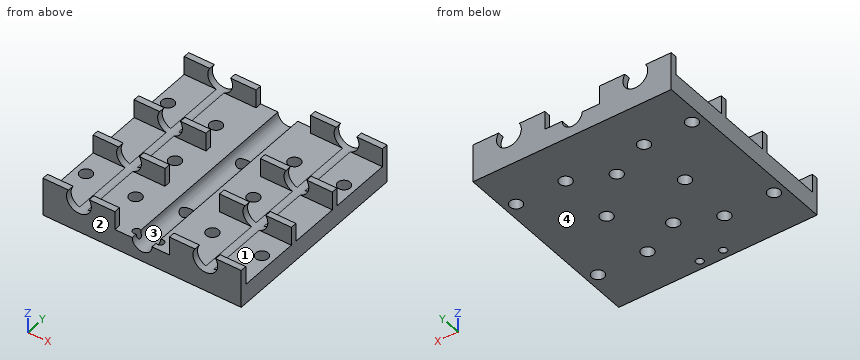
from build123d import *

# Parameters (mm, degrees)
F0_W     = 80
F0_H     = 80
F0_R     = 2.5
F0_R_2   = 1.5
F1_DEPTH = 8
F2_W     = 29
F2_H     = 2.5
F3_DEPTH = 7.5
F5_D     = 10
F7_D     = 8


with BuildPart() as f1:
    # F0 (on Top) → F1 (new body)
    with BuildSketch(Plane.XY):
        Rectangle(F0_W, F0_H)
        with Locations((-35.5, -22.5)):
            Circle(F0_R, mode=Mode.SUBTRACT)
        with Locations((-4.75, -36.5)):
            Circle(F0_R_2, mode=Mode.SUBTRACT)
        with Locations((-15.5, -22.5)):
            Circle(F0_R, mode=Mode.SUBTRACT)
        with Locations((4.75, -36.5)):
            Circle(F0_R_2, mode=Mode.SUBTRACT)
        with Locations((15.5, -22.5)):
            Circle(F0_R, mode=Mode.SUBTRACT)
        with Locations((35.5, -22.5)):
            Circle(F0_R, mode=Mode.SUBTRACT)
        with Locations((0, -15.5)):
            Circle(F0_R, mode=Mode.SUBTRACT)
        with Locations((-16.135083, 0)):
            Circle(F0_R, mode=Mode.SUBTRACT)
        with Locations((-35.5, 22.5)):
            Circle(F0_R, mode=Mode.SUBTRACT)
        with Locations((-16.135083, 22.5)):
            Circle(F0_R, mode=Mode.SUBTRACT)
        with Locations((15.5, 0)):
            Circle(F0_R, mode=Mode.SUBTRACT)
        with Locations((0, 15.5)):
            Circle(F0_R, mode=Mode.SUBTRACT)
        with Locations((15.5, 22.5)):
            Circle(F0_R, mode=Mode.SUBTRACT)
        with Locations((35.5, 22.5)):
            Circle(F0_R, mode=Mode.SUBTRACT)
    extrude(amount=F1_DEPTH)

    # F2 (on face) → F3 (join)
    with BuildSketch(Plane.XY.offset(8)):
        with Locations((-25.5, 38.75)):
            Rectangle(F2_W, F2_H)
        with Locations((25.5, 38.75)):
            Rectangle(F2_W, F2_H)
        with Locations((-25.5, -38.75)):
            Rectangle(F2_W, F2_H)
        with Locations((25.5, -38.75)):
            Rectangle(F2_W, F2_H)
        with Locations((-25.5, -11.25)):
            Rectangle(F2_W, F2_H)
        with Locations((25.5, -11.25)):
            Rectangle(F2_W, F2_H)
        with Locations((-25.5, 11.25)):
            Rectangle(F2_W, F2_H)
        with Locations((25.5, 11.25)):
            Rectangle(F2_W, F2_H)
    extrude(amount=F3_DEPTH)

    # F5 (through all)
    with Locations(Plane(origin=(0, 40, 0), x_dir=(-1, 0, 0), z_dir=(0, 1, 0))):
        with Locations((-25.5, 12.75), (25.5, 12.75)):
            Hole(F5_D / 2)

    # F7 (through all)
    with Locations(Plane(origin=(0, 40, 0), x_dir=(-1, 0, 0), z_dir=(0, 1, 0))):
        with Locations((0, 8)):
            Hole(F7_D / 2)


solid = f1.part
The listing builds one solid part. Answer for the finished solid, in the listing's coordinates (mm). Face numbers are marked on the shaded views. A direction names the side the tool comes from. Round coordinates to 2 decimals unless told otherwise and drop trailing zeros. Write each loop counter-clockwise with the first axis right and the second up, starting at its lowest first coordinate (ties: lowest second). Pieces come first, ordered by that corner, then holes. Notation, with made-up numbers: (47.5, 17) - (66.5, 17) arc R32 cw to (66.5, 44) - close; hole circle Ø6 at (-22, -10). An arc over 180 degrees is marked (long way). Use a Markdown table: item, result. Add a question column.
1. Consider line 1 (Y direction, x = 15.5, z = 4); line 2 (Y direction, x = 18, z = 14.5); line 3 (Y direction, x = 0, z = 2.65). Determine where each line is inside the solid, lowest interval first.
2. The part is cut by section A-A (y = 22.5). Write down the section's boundary in (x, z), and give its area (3 significant figures).
3. The part is cut by section C-C (y = -15.5). Write down the section's boundary in (x, z).
4. The part is cut by section D-D (x = 15.5). Write down the section's boundary in (y, z).
5. A tool of negligible diameter and unlimited length cuts with its end or side. For the marked faces 1 and 2, from which of +Z, -Z, +X, -X, +Y, -Y can it reach the whole face along a straight path? Write none if from no direction.
6. Flat-ended cylindrical pins translate along their axes: P1, Ø3, axis at x = -35.5, y = 22.5, coming from the +Z side; P2, Ø6, axis at x = -16.14, y = 22.5, coming from the +Z side. Find the tip coordinate at first contact, or state that the pin passes through.
7. The part is cut by section B-B (x = 0). Write down the section's boundary in (y, z), and give its area (3 significant figures).
8. For a pull along X with two mould halves and no side action, classify the marked faces 3 and 4 as +X half, -X half, draft (parallel to the pull), parting line (faces both ways), or undercut.
Reported:
| question | item | result |
|---|---|---|
| 1 | line 1 | -40 to -25, -20 to -2.5, 2.5 to 20, 25 to 40 |
| 1 | line 2 | -40 to -37.5, -12.5 to -10, 10 to 12.5, 37.5 to 40 |
| 1 | line 3 | -40 to -18, -13 to 13, 18 to 40 |
| 2 | outline | (-40, 0) - (-38, 0) - (-38, 8) - (-40, 8) - close; (-33, 0) - (-18.64, 0) - (-18.64, 8) - (-23.94, 8) arc R5 cw to (-27.06, 8) - (-33, 8) - close; (-13.64, 0) - (13, 0) - (13, 8) - (4, 8) arc R4 cw to (-4, 8) - (-13.64, 8) - close; (18, 0) - (33, 0) - (33, 8) - (27.06, 8) arc R5 cw to (23.94, 8) - (18, 8) - close; (38, 0) - (40, 0) - (40, 8) - (38, 8) - close |
| 2 | area | 454 mm^2 |
| 3 | outline | (-40, 0) - (-2.5, 0) - (-2.5, 4.88) arc R4 cw to (-4, 8) - (-23.94, 8) arc R5 cw to (-27.06, 8) - (-40, 8) - close; (2.5, 0) - (40, 0) - (40, 8) - (27.06, 8) arc R5 cw to (23.94, 8) - (4, 8) arc R4 cw to (2.5, 4.88) - close |
| 4 | outline | (-40, 0) - (-25, 0) - (-25, 8) - (-37.5, 8) - (-37.5, 15.5) - (-40, 15.5) - close; (-20, 0) - (-2.5, 0) - (-2.5, 8) - (-10, 8) - (-10, 15.5) - (-12.5, 15.5) - (-12.5, 8) - (-20, 8) - close; (2.5, 0) - (20, 0) - (20, 8) - (12.5, 8) - (12.5, 15.5) - (10, 15.5) - (10, 8) - (2.5, 8) - close; (25, 0) - (40, 0) - (40, 15.5) - (37.5, 15.5) - (37.5, 8) - (25, 8) - close |
| 5 | face 1 | +Z, +X, -X |
| 5 | face 2 | +Z, -Z, +X, -X, -Y |
| 6 | P1 | through |
| 6 | P2 | z = 8 |
| 7 | outline | (-40, 0) - (-18, 0) - (-18, 4) - (-40, 4) - close; (-13, 0) - (13, 0) - (13, 4) - (-13, 4) - close; (18, 0) - (40, 0) - (40, 4) - (18, 4) - close |
| 7 | area | 280 mm^2 |
| 8 | face 3 | undercut |
| 8 | face 4 | draft |
